```python
from build123d import *

# Parameters (mm, degrees)
SKETCH1_W                    = 136
SKETCH1_H                    = 198
BASE_FLANGE1_DEPTH           = 1
EDGE_FLANGE1_STRIP_W         = 6
EDGE_FLANGE1_STRIP_H         = 1
EDGE_FLANGE1_STRIP_CUT_DEPTH = 136
EDGE_FLANGE1_DEPTH           = 136
EDGE_FLANGE2_DEPTH           = 197
EDGE_FLANGE3_DEPTH           = 197
CUT_EXTRUDE1_DEPTH           = 515.988593157
CUT_EXTRUDE1_DEPTH_BACK      = 159
SKETCH18_R                   = 1.5
SKETCH21_R                   = 2.25
CUT_EXTRUDE2_DEPTH           = 278
SKETCH26_R                   = 1.5
CUT_EXTRUDE7_DEPTH           = 10
SKETCH33_R                   = 1.55
CUT_EXTRUDE14_DEPTH          = 10


# Sheet-metal steps are written as plain solids
with BuildPart() as part:
    # Sketch1 → Base-Flange1 (new body)
    with BuildSketch(Plane(origin=(0, 0, 0), x_dir=(1, 0, 0), z_dir=(0, 1, 0))):
        with Locations((68, 99)):
            Rectangle(SKETCH1_W, SKETCH1_H)
    extrude(amount=-BASE_FLANGE1_DEPTH)

    # Edge-Flange1 strip (across the edge) → Edge-Flange1 strip cut (cut)
    with BuildSketch(Plane(origin=(136, 0, -198), x_dir=(0, 0, 1), z_dir=(-1, 0, 0))):
        with Locations((-2, -0.5)):
            Rectangle(EDGE_FLANGE1_STRIP_W, EDGE_FLANGE1_STRIP_H)
    extrude(amount=EDGE_FLANGE1_STRIP_CUT_DEPTH, mode=Mode.SUBTRACT)

    # Edge-Flange1 section (across the edge) → Edge-Flange1 (add)
    with BuildSketch(Plane(origin=(136, 0, -198), x_dir=(0, 0, 1), z_dir=(-1, 0, 0))):
        with BuildLine():
            Line((-1, 1), (-1, 19))
            Line((-1, 19), (0, 19))
            Line((0, 19), (0, 1))
            ThreePointArc((0, 1), (0.292893219, 0.292893219), (1, 0))
            Line((1, 0), (1, -1))
            ThreePointArc((1, -1), (-0.414213562, -0.414213562), (-1, 1))
        make_face()
    extrude(amount=EDGE_FLANGE1_DEPTH)

    # Edge-Flange2 section (across the edge) → Edge-Flange2 (add)
    with BuildSketch(Plane(origin=(137, 0, 0), x_dir=(-1, 0, 0), z_dir=(0, 0, -1))):
        with BuildLine():
            Line((-1, 1), (-1, 19))
            Line((-1, 19), (0, 19))
            Line((0, 19), (0, 1))
            ThreePointArc((0, 1), (0.292893219, 0.292893219), (1, 0))
            Line((1, 0), (1, -1))
            ThreePointArc((1, -1), (-0.414213562, -0.414213562), (-1, 1))
        make_face()
    extrude(amount=EDGE_FLANGE2_DEPTH)

    # Edge-Flange3 section (across the edge) → Edge-Flange3 (add)
    with BuildSketch(Plane(origin=(-1, 0, -197), x_dir=(1, 0, 0), z_dir=(0, 0, 1))):
        with BuildLine():
            Line((-1, 1), (-1, 19))
            Line((-1, 19), (0, 19))
            Line((0, 19), (0, 1))
            ThreePointArc((0, 1), (0.292893219, 0.292893219), (1, 0))
            Line((1, 0), (1, -1))
            ThreePointArc((1, -1), (-0.414213562, -0.414213562), (-1, 1))
        make_face()
    extrude(amount=EDGE_FLANGE3_DEPTH)

    # Sketch18 → Cut-Extrude1 (cut, two sides: drawn at the far end of the back side and taken through both)
    with BuildSketch(Plane(origin=(-3, 352.051657269, -347.400026456), x_dir=(0, 0, -1), z_dir=(-1, 0, 0)).offset(-CUT_EXTRUDE1_DEPTH_BACK)):
        with Locations(Location((-298.400026456, 343.051657269, 0), (0, 0, 270))):
            Circle(SKETCH18_R)
        with Locations(Location((-198.400026456, 343.051657269, 0), (0, 0, 270))):
            Circle(SKETCH18_R)
    extrude(amount=CUT_EXTRUDE1_DEPTH + CUT_EXTRUDE1_DEPTH_BACK, mode=Mode.SUBTRACT)

    # Sketch21 → Cut-Extrude2 (cut)
    with BuildSketch(Plane(origin=(-57.062536038, -1, -347.400026456), x_dir=(0, 0, 1), z_dir=(0, -1, 0))):
        with Locations(Location((339.900026456, -95.062536038, 0), (0, 0, 180))):
            Circle(SKETCH21_R)
        with Locations(Location((339.900026456, -155.062536038, 0), (0, 0, 180))):
            Circle(SKETCH21_R)
    extrude(amount=-CUT_EXTRUDE2_DEPTH, mode=Mode.SUBTRACT)

    # Sketch26 → Cut-Extrude7 (cut)
    with BuildSketch(Plane(origin=(-57.062536038, 352.051657269, -200), x_dir=(1, 0, 0), z_dir=(0, 0, -1))):
        with Locations(Location((105.062536038, 343.051657269, 0), (0, 0, 90))):
            Circle(SKETCH26_R)
        with Locations(Location((145.062536038, 343.051657269, 0), (0, 0, 90))):
            Circle(SKETCH26_R)
    extrude(amount=-CUT_EXTRUDE7_DEPTH, mode=Mode.SUBTRACT)

    # Sketch33 → Cut-Extrude14 (cut)
    with BuildSketch(Plane(origin=(193.062536038, -94.051657269, -200), x_dir=(-1, 0, 0), z_dir=(0, 0, -1))):
        with Locations(Location((145.062536038, 103.051657269, 0), (0, 0, 270))):
            Circle(SKETCH33_R)
    extrude(amount=-CUT_EXTRUDE14_DEPTH, mode=Mode.SUBTRACT)


solid = part.part
```
Model file for the job. Use its own axes, mm. A direction names the side the tool comes from. Coordinates: 2 decimals unless noted, no trailing zeros. Write each loop counter-clockwise with the first axis right and the second up, starting at its lowest first coordinate (ties: lowest second). Pieces come first, ordered by that corner, then holes. Notation, with made-up numbers: (-33, -19.75) - (26, -19.75) arc R23 cw to (26, -9.75) - close; hole circle Ø2 at (-25, -24.75). An arc over 180 degrees is marked (long way). One line per item, written item: value. Start each with the question number.
1. Slice it at B-B (y = 14.25). Write the cut outline in (x, z).
2. Slice it at D-D (z = -63). Write the cut outline in (x, y), plus the area to 3 significant figures.
3. Probe line 1 (Z direction, x = 137.7, y = 9); line 2 (X direction, y = 12.25, z = -122.5); line 3 (Z direction, x = 74, y = 15). List the from-to ranges inside material, lowest first. Write a range as from..to.
4. Tool access for faces 1 (the flat face through (67, 0, -100)), 2 (the flat face through (69, 10, -198)), 3 (the flat face through (137, 10, -97)): list every direction of +Z, -Z, +X, -X, +Y, -Y with a clear straight run to the whole face (end or side of a thin tool).
5. Mould opens along X. For faces 4 (the flat face through (68.3, -0.6, 0)), 5 (the flat face through (-2, 10, -100)), 6 (the flat face through (-1, 10, -100)), 7 (the cylindrical face through (95.804, -0.507, -7.012)) say: released by +X, released by -X, zero draft, split by the parting line, or undercut.
6. Slice it at A-A (z = -7.5). Write the cut outline in (x, y), plus the area to 3 significant figures.
7. Flat gauge pins, fed straight in: pin 1 (6 mm diameter, centred on x = 38, z = -7.5, fed in from -Y); pin 2 (6 mm diameter, centred on x = 83.5, z = -164.5, fed in from +Y); pin 3 (1.6 mm diameter, centred on y = 4.5, z = -198.5, fed in from +X); pin 4 (2.5 mm diameter, centred on x = 98, z = -7.5, fed in from -Y). Where does each tip first touch, or does it go through?
8. Slice it at C-C (x = 38). Write the cut outline in (y, z).
Answers below:
1. outline: (-2, -197) - (-1, -197) - (-1, 0) - (-2, 0) - close; (0, -199) - (136, -199) - (136, -198) - (0, -198) - close; (137, -197) - (138, -197) - (138, 0) - (137, 0) - close
2. outline: (-2, 1) arc R2 ccw to (0, -1) - (136, -1) arc R2 ccw to (138, 1) - (138, 19) - (137, 19) - (137, 1) arc R1 cw to (136, 0) - (0, 0) arc R1 cw to (-1, 1) - (-1, 19) - (-2, 19) - close
2. area: 177 mm^2
3. line 1: z = -197..-150.5, -147.5..-50.5, -47.5..0
3. line 2: x = -2..-1, 137..138
3. line 3: z = -199..-198
4. face 1: +Z, +Y
4. face 2: +Z, +X, -X, +Y
4. face 3: +Z, -Z, +Y
5. face 4: zero draft
5. face 5: released by -X
5. face 6: undercut
5. face 7: undercut
6. outline: (-2, 1) arc R2 ccw to (0, -1) - (35.75, -1) - (35.75, 0) - (0, 0) arc R1 cw to (-1, 1) - (-1, 19) - (-2, 19) - close; (40.25, -1) - (95.75, -1) - (95.75, 0) - (40.25, 0) - close; (100.25, -1) - (136, -1) arc R2 ccw to (138, 1) - (138, 19) - (137, 19) - (137, 1) arc R1 cw to (136, 0) - (100.25, 0) - close
6. area: 168 mm^2
7. pin 1: stops at y = -1
7. pin 2: stops at y = 0
7. pin 3: stops at x = 136
7. pin 4: passes through
8. outline: (-1, -197) arc R2 ccw to (1, -199) - (19, -199) - (19, -198) - (1, -198) arc R1 cw to (0, -197) - (0, -9.75) - (-1, -9.75) - close; (-1, -5.25) - (0, -5.25) - (0, 0) - (-1, 0) - close
